```python
from build123d import *

# Parameters (mm, degrees)
SKETCH1_R               = 9.128125
SKETCH1_R_2             = 6.5484375
EXTRUDE1_DEPTH          = 20.6375
CUT_EXTRUDE1_DEPTH      = 10.128125
CUT_EXTRUDE1_DEPTH_BACK = 10.128125


with BuildPart() as part:
    # Sketch1 → Extrude1 (new body)
    with BuildSketch(Plane.XY):
        Circle(SKETCH1_R)
        Circle(SKETCH1_R_2, mode=Mode.SUBTRACT)
    extrude(amount=EXTRUDE1_DEPTH)

    # Sketch2 → Cut-Extrude1 (cut, two sides)
    with BuildSketch(Plane(origin=(0, 0, 0), x_dir=(1, 0, 0), z_dir=(0, 1, 0))) as cut_extrude1_sk:
        with BuildLine():
            Line((-1.190625, -20.6375), (-1.190625, -18.653125))
            ThreePointArc((-1.190625, -18.653125), (0, -17.4625), (1.190625, -18.653125))
            Line((1.190625, -18.653125), (1.190625, -20.6375))
            Line((1.190625, -20.6375), (-1.190625, -20.6375))
        make_face()
    extrude(amount=CUT_EXTRUDE1_DEPTH, mode=Mode.SUBTRACT)
    extrude(cut_extrude1_sk.sketch, amount=-CUT_EXTRUDE1_DEPTH_BACK, mode=Mode.SUBTRACT)


solid = part.part
```
Can you work these out from the model? Positions are in its coordinate system, mm. A direction names the side the tool comes from. Round coordinates to 2 decimals unless told otherwise and drop trailing zeros. Loops run counter-clockwise (first coordinate to the right, second up) from the corner with the lowest first, then second, coordinate; pieces in that order, holes last. Notation, with made-up numbers: M 64,54 L 97,54 A9 ccw 97,71 Z; hole C 1.25,-25 d8. An arc over 180 degrees is marked long. Answer as a JSON object with one key per item and string values. Group by question number.
Q1. Imagine slicing it at B-B, the plane y = 0. Please give me the cut outline in (x, z), then the cut area to 3 significant figures.
Q2. Imagine slicing it at A-A, the plane x = 0. Please give me the cut outline in (y, z).
Q3. We'd pull the mould along Y, two halves only. Please class faces 3 (the flat face through (4, -6, 0)), 4 (the cylindrical face through (-1.42, -6.393, 10.174)), 5 (the cylindrical face through (4.21, -8.1, 10.17)): +Y half, -Y half, draft (parallel to the pull), parting line (faces both ways), or undercut.
Q4. Will these pins go through, and if not, where does the flat tip stop? pin 1 (5 mm diameter, centred on y = 2.5, z = 18, fed in from +X); pin 2 (1.5 mm diameter, centred on y = 3.5, z = 10.5, fed in from -X); pin 3 (0.6 mm diameter, centred on y = -7.5, z = 20, fed in from +X); pin 4 (5 mm diameter, centred on y = 5.5, z = 12.5, fed in from -X).
Q5. Please list where these lines run through material, in increasing order: L1, parallel to Y at x = 0, z = 14.5; L2, parallel to Y at x = 1.5, z = 2.
Q6. Imagine slicing it at C-C, the plane z = 16.75. Please give me the cut outline in (x, y).
Q7. On a 3-axis mill with a long thin cutter (end or side, diameter ignored), from which of +Z, -Z, +X, -X, +Y, -Y can I reach the whole of each face in a straight line? I mean faces 1 (the flat face through (-1.191, -8, 20)), 2 (the flat face through (7, 0, 20.638)). Say none if no direction works.
Findings:
{
 "1": {"outline": "M -9.13,0 L -6.55,0 L -6.55,20.64 L -9.13,20.64 Z; M 6.55,0 L 9.13,0 L 9.13,20.64 L 6.55,20.64 Z", "area": "106 mm2"},
 "2": {"outline": "M -9.13,0 L -6.55,0 L -6.55,17.46 L -9.13,17.46 Z; M 6.55,0 L 9.13,0 L 9.13,17.46 L 6.55,17.46 Z"},
 "3": {"face 3": "draft", "face 4": "undercut", "face 5": "parting line"},
 "4": {"pin 1": "stops at x = 9.13", "pin 2": "stops at x = -8.7", "pin 3": "stops at x = 5.61", "pin 4": "stops at x = -8.62"},
 "5": {"L1": "y = -9.13 to -6.55, 6.55 to 9.13", "L2": "y = -9 to -6.37, 6.37 to 9"},
 "6": {"outline": "C 0,0 d18.26; hole C 0,0 d13.1"},
 "7": {"face 1": "+Z, +Y, -Y", "face 2": "+Z, +X, -X, +Y, -Y"}
}
